Could you check a few things on this drawing? It's one solid part, dimensions in mm from its lowest x, y, z. A direction names the side the tool comes from. Give positions to 0.01 mm unless a question says otherwise; leave off trailing zeros. Write each loop counter-clockwise with the first axis right and the second up, starting at its lowest first coordinate (ties: lowest second). Pieces come first, ordered by that corner, then holes. Notation, with made-up numbers: M -37,79.5 L 2,79.5 A15 ccw 2,86.5 Z; hole C 57,27.5 d7. An arc over 180 degrees is marked long. Answer as CSV lines item,"result". Start each with the question number.
Q1. Suppose I cut it at B-B (x = 38). Write out the boundary of the cut face in (y, z) (1 decimal).
Q2. Thinking about a two-plate mould opening in Z: for the marked faces 1, 2, 3 and 4, which applies, +Z half, -Z half, draft (parallel to the pull), parting line (faces both ways), or undercut?
Q3. Suppose I cut it at C-C (y = 18). Write out the boundary of the cut face in (x, z), then the cut area to 3 significant figures.
Q4. For pin 1 (4 mm diameter, centred on y = 5.5, z = 30, fed in from -X); pin 2 (5 mm diameter, centred on x = 72.5, z = 52, fed in from -Y), each with a flat end and sliding along its axis, tell me the tip position at first contact or that it passes through.
Q5. On a 3-axis mill with a long thin cutter (end or side, diameter ignored), from which of +Z, -Z, +X, -X, +Y, -Y can I reach the whole of each face in a straight line? I mean the marked faces 5 and 6. Say none if no direction works.
Q6. Suppose I cut it at D-D (x = 20.5). Write out the boundary of the cut face in (y, z), then the cut area to 3 significant figures.
Q7. Suppose I cut it at A-A (z = 39.5). Write out the boundary of the cut face in (x, y) (1 decimal), then the cut area to 3 significant figures.
Q8. If I drill on line 1 along Z through (x, y) = (41.5, 23); line 2 along Y through (x, z) = (46, 8); line 3 along X through (y, z) = (12, 26.5) (1 decimal), over which ranges is the centre line in solid material (lowest first)?
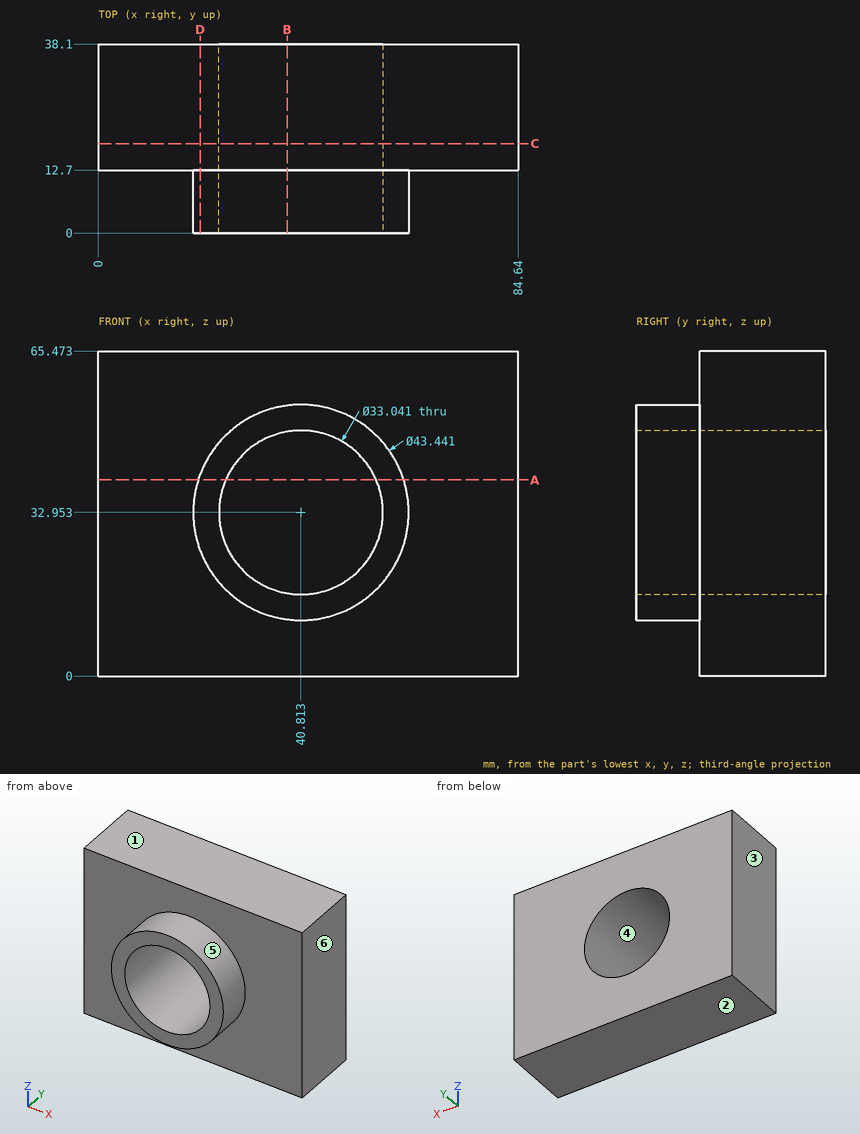
Resolved:
1,outline,"M 0,11.4 L 12.7,11.4 L 12.7,0 L 38.1,0 L 38.1,16.7 L 0,16.7 Z; M 0,49.2 L 38.1,49.2 L 38.1,65.5 L 12.7,65.5 L 12.7,54.5 L 0,54.5 Z"
2,face 1,"+Z half"
2,face 2,"-Z half"
2,face 3,"draft"
2,face 4,"undercut"
3,outline,"M 0,0 L 84.64,0 L 84.64,65.47 L 0,65.47 Z; hole C 40.81,32.95 d33.04"
3,area,"4,680 mm^2"
4,pin 1,"x = 19.11"
4,pin 2,"y = 12.7"
5,face 5,"-Y"
5,face 6,"+Z, -Z, +X, +Y, -Y"
6,outline,"M 0,25.26 L 12.7,25.26 L 12.7,0 L 38.1,0 L 38.1,65.47 L 12.7,65.47 L 12.7,40.65 L 0,40.65 Z"
6,area,"1,860 mm^2"
7,outline,"M 0,12.7 L 20.1,12.7 L 20.1,0 L 25.6,0 L 25.6,38.1 L 0,38.1 Z; M 56,0 L 61.5,0 L 61.5,12.7 L 84.6,12.7 L 84.6,38.1 L 56,38.1 Z"
7,area,"1,520 mm^2"
8,line 1,"0 to 16.45, 49.46 to 65.47"
8,line 2,"12.7 to 38.1"
8,line 3,"20.1 to 25.6, 56 to 61.6"
